```python
from build123d import *

# Parameters (mm, degrees)
F0_W     = 76.2
F0_H     = 127
F1_DEPTH = 88.9
F2_W     = 63.5
F2_H     = 114.3
F3_DEPTH = 82.55
F4_R     = 18.190192
F5_DEPTH = 76.201


with BuildPart() as f1:
    # F0 (on Top) → F1 (new body)
    with BuildSketch(Plane.XY):
        Rectangle(F0_W, F0_H)
    extrude(amount=F1_DEPTH)

    # F2 (on face) → F3 (cut)
    with BuildSketch(Plane.XY.offset(88.9)):
        Rectangle(F2_W, F2_H)
    extrude(amount=-F3_DEPTH, mode=Mode.SUBTRACT)

    # F4 (on face) → F5 (cut, through all)
    with BuildSketch(Plane.YZ.offset(38.1)):
        with Locations((-25.125185, 53.211018)):
            Circle(F4_R)
    extrude(amount=-F5_DEPTH, mode=Mode.SUBTRACT)


solid = f1.part
```
The listing builds one solid part. Answer for the finished solid, in the listing's coordinates (mm). A direction names the side the tool comes from. Round coordinates to 2 decimals unless told otherwise and drop trailing zeros. Loops run counter-clockwise (first coordinate to the right, second up) from the corner with the lowest first, then second, coordinate; pieces in that order, holes last. Notation, with made-up numbers: (45.25, 57.25) - (75.25, 57.25) arc R12 cw to (75.25, 67.25) - close; hole circle Ø5 at (-10.5, 5). An arc over 180 degrees is marked (long way). Return JSON: item names as keys, results as strings. Group by question number.
1. The mould has two halves that part along X. Classify faces 1 (the flat face through (0, 1, 6.35)), 2 (the flat face through (38.1, -1, 44)), 3 (the flat face through (-38.1, -1, 44)): pulls with the +X half, pulls with the -X half, needs draft (parallel to the pull), parting line crosses it, or undercut.
2. Consider probe 1 along Y at (x, z) = (-14, 68); probe 2 along X at (y, z) = (-8, 68). Determine where each line is inside the solid, lowest interval first.
3. Which of the six approach directions +Z, -Z, +X, -X, +Y, -Y give full straight-line access (tool end or side, diameter ignored) to faces 4 (the flat face through (-34, 5, 88.9)), 5 (the flat face through (0, 57.15, 48))?
4. This flat-tipped pin is pushed along its axis until it touches: P1, Ø4, axis at x = -19, y = -10.5, coming from the +Z side. Where does it stop, or does it pass through?
5. The part is cut by section A-A on z = 57. Determine the outline of the cut face in (x, y), then the cut area to 3 significant figures.
6. The part is cut by section C-C on x = 18. Determine the outline of the cut face in (y, z), then the cut area to 3 significant figures.
7. The part is cut by section B-B on y = -23. Determine the outline of the cut face in (x, z), then the cut area to 3 significant figures.
8. The part is cut by section D-D on z = 29. Determine the outline of the cut face in (x, y), then the cut area to 3 significant figures.
Resolved:
{
 "1": {"face 1": "undercut", "face 2": "pulls with the +X half", "face 3": "pulls with the -X half"},
 "2": {"probe 1": "y = -63.5 to -57.15, 57.15 to 63.5", "probe 2": "x = -38.1 to -31.75, 31.75 to 38.1"},
 "3": {"face 4": "+Z, +X, -X, +Y, -Y", "face 5": "+Z"},
 "4": {"P1": "stops at z = 6.35"},
 "5": {"outline": "(-38.1, -63.5) - (38.1, -63.5) - (38.1, -42.92) - (31.75, -42.92) - (31.75, -57.15) - (-31.75, -57.15) - (-31.75, -42.92) - (-38.1, -42.92) - close; (-38.1, -7.33) - (-31.75, -7.33) - (-31.75, 57.15) - (31.75, 57.15) - (31.75, -7.33) - (38.1, -7.33) - (38.1, 63.5) - (-38.1, 63.5) - close", "area": "1,970 mm²"},
 "6": {"outline": "(-63.5, 0) - (63.5, 0) - (63.5, 88.9) - (57.15, 88.9) - (57.15, 6.35) - (-57.15, 6.35) - (-57.15, 88.9) - (-63.5, 88.9) - close", "area": "1,850 mm²"},
 "7": {"outline": "(-38.1, 0) - (38.1, 0) - (38.1, 35.15) - (31.75, 35.15) - (31.75, 6.35) - (-31.75, 6.35) - (-31.75, 35.15) - (-38.1, 35.15) - close; (-38.1, 71.28) - (-31.75, 71.28) - (-31.75, 88.9) - (-38.1, 88.9) - close; (31.75, 71.28) - (38.1, 71.28) - (38.1, 88.9) - (31.75, 88.9) - close", "area": "1,070 mm²"},
 "8": {"outline": "(-38.1, -63.5) - (38.1, -63.5) - (38.1, 63.5) - (-38.1, 63.5) - close; hole (-31.75, -57.15) - (31.75, -57.15) - (31.75, 57.15) - (-31.75, 57.15) - close", "area": "2,420 mm²"}
}
